Input: part model. Units: mm. Frame: model coordinates. Face numbers are marked on the shaded views. A direction names the side the tool comes from. Round coordinates to 2 decimals unless told otherwise and drop trailing zeros. Write each loop counter-clockwise with the first axis right and the second up, starting at its lowest first coordinate (ties: lowest second). Pieces come first, ordered by that corner, then holes. Notation, with made-up numbers: (70, 26.25) -> (75, 26.25) arc R24 ccw to (75, 38.25) -> close; hole circle Ø11 at (-16.75, 15). An arc over 180 degrees is marked (long way). Use CSV: the item, a comma, the result in double quotes.
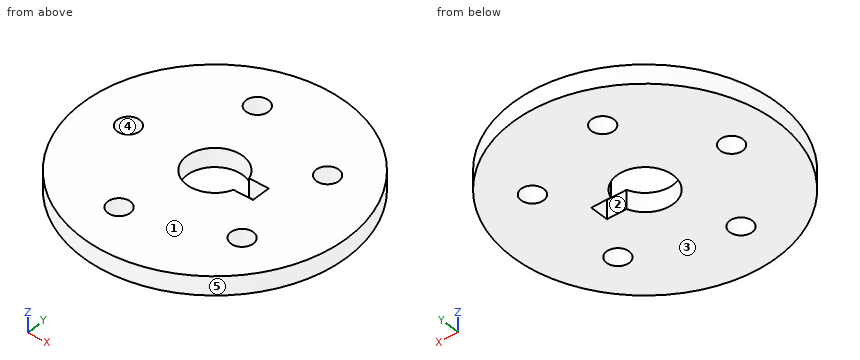
Autodesk Inventor part; units mm, degrees
ref_plane "YZ Plane" through (0, 0, 0) normal (1, 0, 0) x (0, 1, 0)
ref_plane "XZ Plane" through (0, 0, 0) normal (0, 1, 0) x (-1, 0, 0)
ref_plane "XY Plane" through (0, 0, 0) normal (0, 0, 1) x (1, 0, 0)
sketch "Sketch1" plane through (0, 0, 0) normal (0, 0, 1) x (1, 0, 0)
  line L0 (-25.1788, 61.8531) -> (-25.1788, 68.2031)
  line L1 (-13.5921, 60.3277) -> (-11.9486, 66.4613)
  line L2 (-2.7951, 55.8554) -> (0.3799, 61.3547)
  line L3 (6.4766, 48.741) -> (10.9667, 53.2312)
  line L4 (13.591, 39.4694) -> (19.0902, 42.6444)
  line L5 (18.0633, 28.6723) -> (24.1969, 30.3158)
  line L6 (19.5887, 17.0856) -> (25.9387, 17.0856)
  line L7 (18.0633, 5.4989) -> (24.1969, 3.8554)
  line L8 (13.591, -5.2981) -> (19.0902, -8.4731)
  line L9 (6.4766, -14.5698) -> (10.9667, -19.0599)
  line L10 (-2.7951, -21.6842) -> (0.3799, -27.1834)
  line L11 (-13.5921, -26.1565) -> (-11.9486, -32.2901)
  line L12 (-25.1788, -27.6819) -> (-25.1788, -34.0319)
  line L13 (-36.7655, -26.1565) -> (-38.409, -32.2901)
  line L14 (-47.5626, -21.6842) -> (-50.7376, -27.1834)
  line L15 (-56.8342, -14.5698) -> (-61.3243, -19.0599)
  line L16 (-63.9486, -5.2981) -> (-69.4479, -8.4731)
  line L17 (-68.4209, 5.4989) -> (-74.5545, 3.8554)
  line L18 (-69.9463, 17.0856) -> (-76.2963, 17.0856)
  line L19 (-68.4209, 28.6723) -> (-74.5545, 30.3158)
  line L20 (-63.9486, 39.4694) -> (-69.4479, 42.6444)
  line L21 (-56.8342, 48.741) -> (-61.3243, 53.2312)
  line L22 (-47.5626, 55.8554) -> (-50.7376, 61.3547)
  line L23 (-36.7655, 60.3277) -> (-38.409, 66.4613)
  arc A0 (-38.409, 66.4613) -> (-25.1788, 68.2031) centre (-31.8994, 68.1336) ccw
  arc A1 (-25.1788, 68.2031) -> (-11.9486, 66.4613) centre (-18.4582, 68.1336) ccw
  arc A2 (-11.9486, 66.4613) -> (0.3799, 61.3547) centre (-5.475, 64.6547) ccw
  arc A3 (0.3799, 61.3547) -> (10.9667, 53.2312) centre (6.1654, 57.9342) ccw
  arc A4 (10.9667, 53.2312) -> (19.0902, 42.6444) centre (15.6697, 48.4298) ccw
  arc A5 (19.0902, 42.6444) -> (24.1969, 30.3158) centre (22.3903, 36.7894) ccw
  arc A6 (24.1969, 30.3158) -> (25.9387, 17.0856) centre (25.8692, 23.8062) ccw
  arc A7 (25.9387, 17.0856) -> (24.1969, 3.8554) centre (25.8692, 10.365) ccw
  arc A8 (24.1969, 3.8554) -> (19.0902, -8.4731) centre (22.3903, -2.6182) ccw
  arc A9 (19.0902, -8.4731) -> (10.9667, -19.0599) centre (15.6697, -14.2586) ccw
  arc A10 (10.9667, -19.0599) -> (0.3799, -27.1834) centre (6.1654, -23.7629) ccw
  arc A11 (0.3799, -27.1834) -> (-11.9486, -32.2901) centre (-5.475, -30.4835) ccw
  arc A12 (-11.9486, -32.2901) -> (-25.1788, -34.0319) centre (-18.4582, -33.9623) ccw
  arc A13 (-25.1788, -34.0319) -> (-38.409, -32.2901) centre (-31.8994, -33.9623) ccw
  arc A14 (-38.409, -32.2901) -> (-50.7376, -27.1834) centre (-44.8826, -30.4835) ccw
  arc A15 (-50.7376, -27.1834) -> (-61.3243, -19.0599) centre (-56.523, -23.7629) ccw
  arc A16 (-61.3243, -19.0599) -> (-69.4479, -8.4731) centre (-66.0273, -14.2586) ccw
  arc A17 (-69.4479, -8.4731) -> (-74.5545, 3.8554) centre (-72.7479, -2.6182) ccw
  arc A18 (-74.5545, 3.8554) -> (-76.2963, 17.0856) centre (-76.2268, 10.365) ccw
  arc A19 (-76.2963, 17.0856) -> (-74.5545, 30.3158) centre (-76.2268, 23.8062) ccw
  arc A20 (-74.5545, 30.3158) -> (-69.4479, 42.6444) centre (-72.7479, 36.7894) ccw
  arc A21 (-69.4479, 42.6444) -> (-61.3243, 53.2312) centre (-66.0273, 48.4298) ccw
  arc A22 (-61.3243, 53.2312) -> (-50.7376, 61.3547) centre (-56.523, 57.9342) ccw
  arc A23 (-50.7376, 61.3547) -> (-38.409, 66.4613) centre (-44.8826, 64.6547) ccw
  circle A24 centre (-25.1788, 17.0856) radius 44.7675
  point P0 (0, 0)
  dimension "d36" = 89.535
  dimension "d8" = 360
extrude "Extrusion1" add sketch "Sketch1" along normal blind 6.35 contours A24
sketch "Sketch2" plane through (-25.1788, 17.0856, 0) normal (0, 0, -1) x (-1, 0, 0)
  circle A0 centre (-23.7729, 17.272) radius 3.81
  circle A1 centre (0, 0) radius 44.7675
  circle A2 centre (9.0804, 27.9467) radius 3.81
  circle A3 centre (29.3849, 0) radius 3.81
  circle A4 centre (9.0804, -27.9467) radius 3.81
  circle A5 centre (-23.7729, -17.272) radius 3.81
  point P0 (-25.1788, -17.0856)
  dimension "d15" = 360
  dimension "d17" = 17.272
  dimension "d19" = 0
  dimension "d20" = 7.62
hole "Hole1" at (-1.4059, 34.3576, 0) at (-1.4059, -0.1864, 0) at (-34.2592, 45.0323, 0) at (-34.2592, -10.8611, 0) at (-54.5637, 17.0856, 0) direction (0, 0, 1) diameter 7.62 end through all
sketch "Sketch3" plane through (-25.1788, 17.0856, 0) normal (0, 0, -1) x (-1, 0, 0)
  point P0 (-25.1788, -17.0856)
sketch "Sketch4" plane through (-25.1788, 17.0856, 0) normal (0, 0, -1) x (-1, 0, 0)
  point P0 (-25.1788, -17.0856)
sketch "Sketch5" plane through (-25.1788, 17.0856, 6.35) normal (0, 0, 1) x (1, 0, 0)
  arc A0 (8.9803, 3.175) -> (8.9803, -3.175) centre (0, 0) ccw
  line L0 (15.6281, 3.175) -> (8.9803, 3.175)
  line L1 (8.9803, -3.175) -> (15.6281, -3.175)
  line L2 (15.6281, -3.175) -> (15.6281, 3.175)
  circle A1 centre (0, 0) radius 44.7675
  point P0 (25.1788, -17.0856)
  dimension "d28" = 19.05
  dimension "d40" = 0
  dimension "d41" = 6.35
  dimension "d42" = 3.175
  dimension "d43" = 0
  dimension "d46" = 15.6281
extrude "Extrusion2" cut sketch "Sketch5" against normal through all contours L0 L2 L1 A0
properties part number "Seeder Motor Gear"
Item 1: Section query B-B on y = 25.5. Return the cut outline in (x, z).
Worked answers:
outline,"(-69.15, 0) -> (-29.64, 0) -> (-29.64, 6.35) -> (-69.15, 6.35) -> close; (-20.72, 0) -> (18.79, 0) -> (18.79, 6.35) -> (-20.72, 6.35) -> close"
Item 2: First-contact query: pin 1 Ø7 at (x, y) = (-54.56, 17.09) entering from +Z; pin 2 Ø1 at (x, z) = (-32.5, 5.5) entering from +Y; pin 3 Ø9 at (x, y) = (-34.26, 45.03) entering from -Z; pin 4 Ø1.5 at (x, z) = (-22, 2.5) entering from +Y. Flat tips, straight axial feed; report the tip coordinate or a pass-through.
Worked answers:
pin 1,"passes through"
pin 2,"stops at y = 61.33"
pin 3,"stops at z = 0"
pin 4,"stops at y = 61.79"
Item 3: Section query C-C on z = 3.25. Return the cut outline in (x, y) (1 decimal).
Worked answers:
outline,"circle Ø89.5 at (-25.2, 17.1); hole circle Ø7.6 at (-54.6, 17.1); hole circle Ø7.6 at (-34.3, -10.9); hole circle Ø7.6 at (-34.3, 45); hole (-16.2, 13.9) -> (-9.6, 13.9) -> (-9.6, 20.3) -> (-16.2, 20.3) arc R9.5 ccw (long way) to start; hole circle Ø7.6 at (-1.4, -0.2); hole circle Ø7.6 at (-1.4, 34.4)"
Item 4: Set-up query: the marked faces 1 and 2. Return all of +Z, -Z, +X, -X, +Y, -Y with unobstructed straight access to the full face (end or side cutting, diameter ignored); none if empty.
Worked answers:
face 1,"+Z, +X, -X, +Y, -Y"
face 2,"+Z, -Z"
Item 5: Line query: line 1 (X direction, y = 18.5, z = 4.5); line 2 (X direction, y = 18, z = 5.5); line 3 (Y direction, x = -3, z = 2). Output: solid intervals per line, ascending.
Worked answers:
line 1,"x = -69.92 to -58.1, -51.03 to -34.6, -9.55 to 19.57"
line 2,"x = -69.94 to -58.26, -50.87 to -34.66, -9.55 to 19.58"
line 3,"y = -21.8 to -3.65, 3.27 to 30.9, 37.82 to 55.97"
Item 6: Section query D-D on y = -22. Return the cut outline in (x, z), plus the area to 3 significant figures.
Worked answers:
outline,"(-47.01, 0) -> (-3.35, 0) -> (-3.35, 6.35) -> (-47.01, 6.35) -> close"
area,"277 mm²"
Item 7: Section query A-A on x = -57. Return the cut outline in (y, z).
Worked answers:
outline,"(-14.4, 0) -> (14.16, 0) -> (14.16, 6.35) -> (-14.4, 6.35) -> close; (20.01, 0) -> (48.57, 0) -> (48.57, 6.35) -> (20.01, 6.35) -> close"
Item 8: Pull-direction query (X, two-part tool) for the marked faces 3, 4 and 5; classes: +X half, -X half, draft (parallel to the pull), parting line (faces both ways), or undercut.
Worked answers:
face 3,"draft"
face 4,"undercut"
face 5,"parting line"
